Check sheet for the modelled part. Datum: model origin and axes. Units: mm. Give positions to 0.01 mm unless a question says otherwise; leave off trailing zeros. Order: outer loops, then holes, each group sorted by start corner. A loop starts at its lowest first (then second) coordinate and runs counter-clockwise, first axis right, second up. Notation, with made-up numbers: M 2.25,-23 L 11.25,-23 A24 cw 11.25,7 Z; hole C 8,22 d9. An arc over 180 degrees is marked long. Return JSON: item names as keys, results as strings. Group by question number.
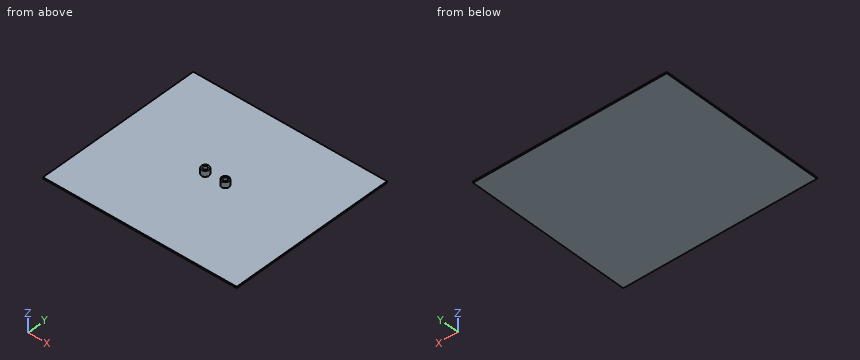
from build123d import *

# Parameters (mm, degrees)
F0_W     = 135.291382
F0_H     = 116.93953
F1_DEPTH = 1
F2_R     = 2.62
F2_R_2   = 1.5
F2_R_3   = 2.6
F3_DEPTH = 4


with BuildPart() as f1:
    # F0 (on Top) → F1 (new body)
    with BuildSketch(Plane.XY):
        Rectangle(F0_W, F0_H)
    extrude(amount=F1_DEPTH)

    # F2 (on face) → F3 (join)
    with BuildSketch(Plane.XY.offset(1)):
        with Locations((-6.825348, 0)):
            Circle(F2_R)
        with Locations((-6.825348, 0)):
            Circle(F2_R_2, mode=Mode.SUBTRACT)
        with Locations((7.174652, 0)):
            Circle(F2_R_3)
        with Locations((7.174652, 0)):
            Circle(F2_R_2, mode=Mode.SUBTRACT)
    extrude(amount=F3_DEPTH)


solid = f1.part
1) Sectioned sample at C-C on x = -50. Record the boundary of the cut face in (y, z).
2) Sectioned sample at D-D on y = 50.5. Record the boundary of the cut face in (x, z), then the cut area to 3 significant figures.
3) Sectioned sample at B-B on y = 0. Record the boundary of the cut face in (x, z).
4) Sectioned sample at A-A on z = 1.9. Record the boundary of the cut face in (x, y), then the cut area to 3 significant figures.
5) Depth check by flat-ended pin: P1, Ø5, axis at x = 7.17, y = 0, coming from the -Z side; P2, Ø1.5, axis at x = -7, y = 0.5, coming from the +Z side. Enter the tip coordinate at first touch or a pass-through.
6) Material ranges on line 1 along Z through (x, y) = (59, 27), recorded low to high.
Reply:
{
 "1": {"outline": "M -58.47,0 L 58.47,0 L 58.47,1 L -58.47,1 Z"},
 "2": {"outline": "M -67.65,0 L 67.65,0 L 67.65,1 L -67.65,1 Z", "area": "135 mm^2"},
 "3": {"outline": "M -67.65,0 L 67.65,0 L 67.65,1 L 9.77,1 L 9.77,5 L 8.67,5 L 8.67,1 L 5.67,1 L 5.67,5 L 4.57,5 L 4.57,1 L -4.21,1 L -4.21,5 L -5.33,5 L -5.33,1 L -8.33,1 L -8.33,5 L -9.45,5 L -9.45,1 L -67.65,1 Z"},
 "4": {"outline": "C -6.83,0 d5.24; C 7.17,0 d5.2; hole C -6.83,0 d3; hole C 7.17,0 d3", "area": "28.7 mm^2"},
 "5": {"P1": "z = 0", "P2": "z = 1"},
 "6": {"line 1": "0 to 1"}
}
